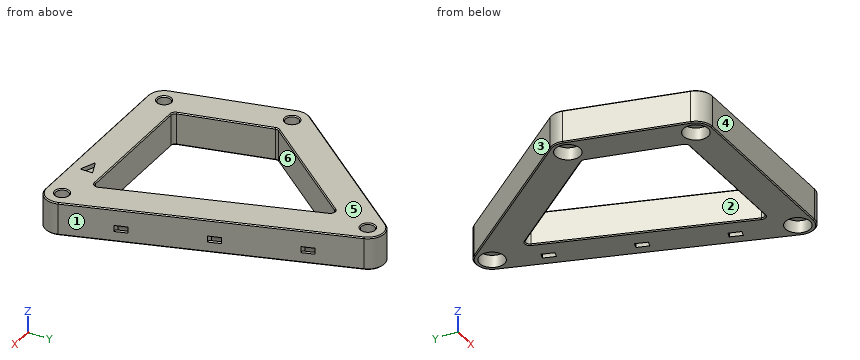
from build123d import *

# Parameters (mm, degrees)
SZKIC1_R                    = 1.55
SZKIC1_R_2                  = 1.6
DODANIE_WYCI_GNI_CIE1_DEPTH = 8
ZAOKR_GLENIE1_R             = 4
SZKIC2_R                    = 3
WYTNIJ_WYCI_GNI_CIE1_DEPTH  = 3
ZAOKR_GLENIE2_R             = 1
SFAZOWANIE1_SIZE            = 0.25
WYTNIJ_WYCI_GNI_CIE2_DEPTH  = 1
WYTNIJ_WYCI_GNI_CIE3_DEPTH  = 3
SZYK_LINIOWY1_COUNT         = 3
SZYK_LINIOWY1_PITCH         = 20


with BuildPart() as part:
    # Szkic1 → Dodanie-wyciągnięcie1 (new body)
    with BuildSketch(Plane.XY):
        Polygon((-32.374614688, -34.065144123), (1.443331859, 8.207289062), (26.5780588, -66), (-24.095207609, -66), align=None)
        with Locations((-21, -62)):
            Circle(SZKIC1_R, mode=Mode.SUBTRACT)
        with Locations((21, -62)):
            Circle(SZKIC1_R, mode=Mode.SUBTRACT)
        Circle(SZKIC1_R_2, mode=Mode.SUBTRACT)
        with Locations((-28, -35)):
            Circle(SZKIC1_R_2, mode=Mode.SUBTRACT)
        Polygon((-23.625385312, -35.934855877), (-1.443331859, -8.207289062), (15.4219412, -58), (-17.904792391, -58), align=None, mode=Mode.SUBTRACT)
    extrude(amount=DODANIE_WYCI_GNI_CIE1_DEPTH)

    # Zaokrąglenie1
    zaokr_glenie1_edges = [part.edges().sort_by_distance(p)[0] for p in [
        (-32.374614688, -34.065144123, 4),
        (1.443331859, 8.207289062, 4),
        (26.5780588, -66, 4),
        (-24.095207609, -66, 4),
    ]]
    fillet(zaokr_glenie1_edges, radius=ZAOKR_GLENIE1_R)

    # Szkic2 → Wytnij-wyciągnięcie1 (cut)
    with BuildSketch(Plane.XY):
        Circle(SZKIC2_R)
        with Locations((-28, -35)):
            Circle(SZKIC2_R)
        with Locations((-21, -62)):
            Circle(SZKIC2_R)
        with Locations((21, -62)):
            Circle(SZKIC2_R)
    extrude(amount=WYTNIJ_WYCI_GNI_CIE1_DEPTH, mode=Mode.SUBTRACT)

    # Zaokrąglenie2
    zaokr_glenie2_edges = [part.edges().sort_by_distance(p)[0] for p in [
        (-23.625385312, -35.934855877, 4),
        (-17.904792391, -58, 4),
        (15.4219412, -58, 4),
        (-1.443331859, -8.207289062, 4),
    ]]
    fillet(zaokr_glenie2_edges, radius=ZAOKR_GLENIE2_R)

    # Sfazowanie1
    sfazowanie1_edges = [part.edges().sort_by_distance(p)[0] for p in [
        (7.058775414, -33.30874863, 0),
        (7.058775414, -33.30874863, 8),
        (-20.799357962, -46.835247082, 0),
        (-20.799357962, -46.835247082, 8),
        (-12.948817041, -22.589145539, 0),
        (-12.948817041, -22.589145539, 8),
        (14.84007865, -57.582749074, 0),
        (14.84007865, -57.582749074, 8),
        (-17.742969998, -57.790873618, 0),
        (-17.742969998, -57.790873618, 8),
        (-23.509651218, -35.959588272, 0),
        (-23.509651218, -35.959588272, 8),
        (-1.630962951, -9.274224983, 0),
        (-1.630962951, -9.274224983, 8),
        (-22.55, -62, 8),
        (19.45, -62, 8),
        (-1.6, 0, 8),
        (-29.6, -35, 8),
        (0, -66, 0),
        (0, -66, 8),
        (-28.371987593, -49.503848635, 0),
        (-17.123475238, -15.00121981, 0),
        (14.288578303, -29.716771865, 0),
        (0.692807492, 3.939545377, 0),
        (24.2506086, -64.330996296, 0),
        (-31.911678313, -34.164073702, 0),
        (-23.44791804, -65.163494471, 0),
        (-28.371987593, -49.503848635, 8),
        (14.288578303, -29.716771865, 8),
        (-17.123475238, -15.00121981, 8),
        (0.692807492, 3.939545377, 8),
        (24.2506086, -64.330996296, 8),
        (-31.911678313, -34.164073702, 8),
        (-23.44791804, -65.163494471, 8),
        (-1.551781994, -58, 0),
        (-1.551781994, -58, 8),
    ]]
    chamfer(sfazowanie1_edges, length=SFAZOWANIE1_SIZE)

    # Szkic3 → Wytnij-wyciągnięcie2 (cut)
    with BuildSketch(Plane(origin=(0, 0, 8), x_dir=(-1, 0, 0), z_dir=(0, 0, -1))):
        Polygon((-11, -60.5), (-11, -63.5), (-7.291900756, -62), align=None)
    extrude(amount=WYTNIJ_WYCI_GNI_CIE2_DEPTH, mode=Mode.SUBTRACT)

    # Szkic4 → Wytnij-wyciągnięcie3 (cut)
    with BuildSketch(Plane(origin=(19.976472797, -46.509603231, 0.25), x_dir=(0.9471445756278131, 0.3208070336803883, 0), z_dir=(-0.3208070336803883, 0.9471445756278131, 0))):
        with BuildLine():
            Line((-4, 0.25), (-2.5, 0.25))
            ThreePointArc((-2.5, 0.25), (-1.767766953, -1.517766953), (0, -2.25))
            Line((0, -2.25), (0, -3.75))
            ThreePointArc((0, -3.75), (-2.828427125, -2.578427125), (-4, 0.25))
        make_face()
    wytnij_wyci_gni_cie3 = extrude(amount=-WYTNIJ_WYCI_GNI_CIE3_DEPTH, mode=Mode.SUBTRACT)

    # Szyk liniowy1: Wytnij-wyciągnięcie3 ×3
    with Locations(*[Vector(-0.3208070336803885, 0.9471445756278131, 0) * (i * SZYK_LINIOWY1_PITCH) for i in range(1, SZYK_LINIOWY1_COUNT)]):
        add(wytnij_wyci_gni_cie3, mode=Mode.SUBTRACT)


solid = part.part
Verification items for the finished model (mm, model axes). Face numbers are marked on the shaded views. A direction names the side the tool comes from. Coordinates: 2 decimals unless noted, no trailing zeros. Order: outer loops, then holes, each group sorted by start corner. A loop starts at its lowest first (then second) coordinate and runs counter-clockwise, first axis right, second up. Notation, with made-up numbers: M 57.25,5 L 100.25,5 A20 ccw 100.25,42 Z; hole C -10,24 d2. An arc over 180 degrees is marked long. One line per item, written item: value. Start each with the question number.
Item 1: Sectioned sample at D-D on z = 1. Give the number of separate pieces and of enclosed holes in the cut face, then the cut area to 3 significant figures.
Item 2: Sectioned sample at B-B on y = -53. Record the cut outline in (x, z), then the cut area to 3 significant figures.
Item 3: Mould release check, pull along Y, two halves, no side actions. Record for the marked faces 3, 4, 5 and 6: pulls with the +Y half, pulls with the -Y half, needs draft (parallel to the pull), parting line crosses it, or undercut.
Item 4: Sectioned sample at C-C on x = -28. Record the cut outline in (y, z).
Item 5: Thickness scan on probe 1 along X at (y, z) = (-35, 5.2); probe 2 along Z at (x, y) = (1, -2); probe 3 along X at (y, z) = (-49.5, 2). Record the ranges inside material, lowest first.
Item 6: Sectioned sample at A-A on z = 5.5. Record the cut outline in (x, y).
Item 7: Depth check by flat-ended pin: P1, Ø3, axis at x = 22, y = -62.5, coming from the -Z side; P2, Ø2.5, axis at x = -28, y = -35, coming from the -Z side; P3, Ø1.5, axis at x = 2, z = 7, coming from the +Y side; P4, Ø4, axis at x = -8, z = 5, coming from the +Y side. Enter the tip coordinate at first touch or a pass-through.
Item 8: Access from +Z, -Z, +X, -X, +Y, -Y to the whole of each face (thin tool, end or side, straight path). Record for the marked faces 1 and 2.
Calculated:
1. separate pieces: 1
1. enclosed holes: 8
1. area: 1,290 mm^2
2. outline: M -27.47,0.25 L -27.21,0 L -19.46,0 L -19.2,0.25 L -19.2,7.75 L -19.46,8 L -27.21,8 L -27.47,7.75 Z; M 13.73,0.25 L 13.99,0 L 21.91,0 L 22.17,0.25 L 22.17,7.75 L 21.91,8 L 13.99,8 L 13.73,7.75 Z
2. area: 133 mm^2
3. face 3: pulls with the +Y half
3. face 4: pulls with the -Y half
3. face 5: needs draft
3. face 6: undercut
4. outline: M -50.94,0.25 L -49.94,0 L -38,0 L -38,3 L -36.6,3 L -36.6,7.75 L -36.85,8 L -49.94,8 L -50.94,7.75 Z; M -33.4,3 L -32,3 L -32,0 L -29,0 L -28.6,0.25 L -28.6,7.75 L -29,8 L -33.15,8 L -33.4,7.75 Z
5. probe 1: -32 to -29.6, -26.4 to -22.88, 7.63 to 16.08
5. probe 2: 3 to 8
5. probe 3: -28.37 to -20.11, 12.54 to 17.33, 19.41 to 20.99
6. outline: M -31.87,-36 L -24.87,-63 A4 ccw -21,-66 L 21,-66 A4 ccw 24.79,-60.72 L 3.79,1.28 A4 ccw -3.12,2.5 L -31.12,-32.5 A4 ccw Z; hole C -28,-35 d3.2; hole M -23.5,-36.42 L -18.1,-57.25 A1 ccw -17.13,-58 L 14.03,-58 A1 ccw 14.97,-56.68 L -0.86,-9.94 A1 ccw -2.59,-9.63 L -23.31,-35.54 A1 ccw Z; hole C -21,-62 d3.1; hole C 0,0 d3.2; hole C 21,-62 d3.1
7. P1: z = 3
7. P2: through
7. P3: y = 3.8
7. P4: y = -1.1
8. face 1: +Z, -Z, +X, +Y
8. face 2: +Z, -Z
